Here's the drawing with two shaded views (mm, measured from the low corner). I have some questions. Give positions to 0.01 mm unless a question says otherwise; leave off trailing zeros. Write each loop counter-clockwise with the first axis right and the second up, starting at its lowest first coordinate (ties: lowest second). Pieces come first, ordered by that corner, then holes. Notation, with made-up numbers: M 18,24 L 49,24 A18 cw 49,43 Z; hole C -11.5,66.25 d1. An arc over 180 degrees is marked long. Answer as CSV lines item,"result". Start each with the question number.
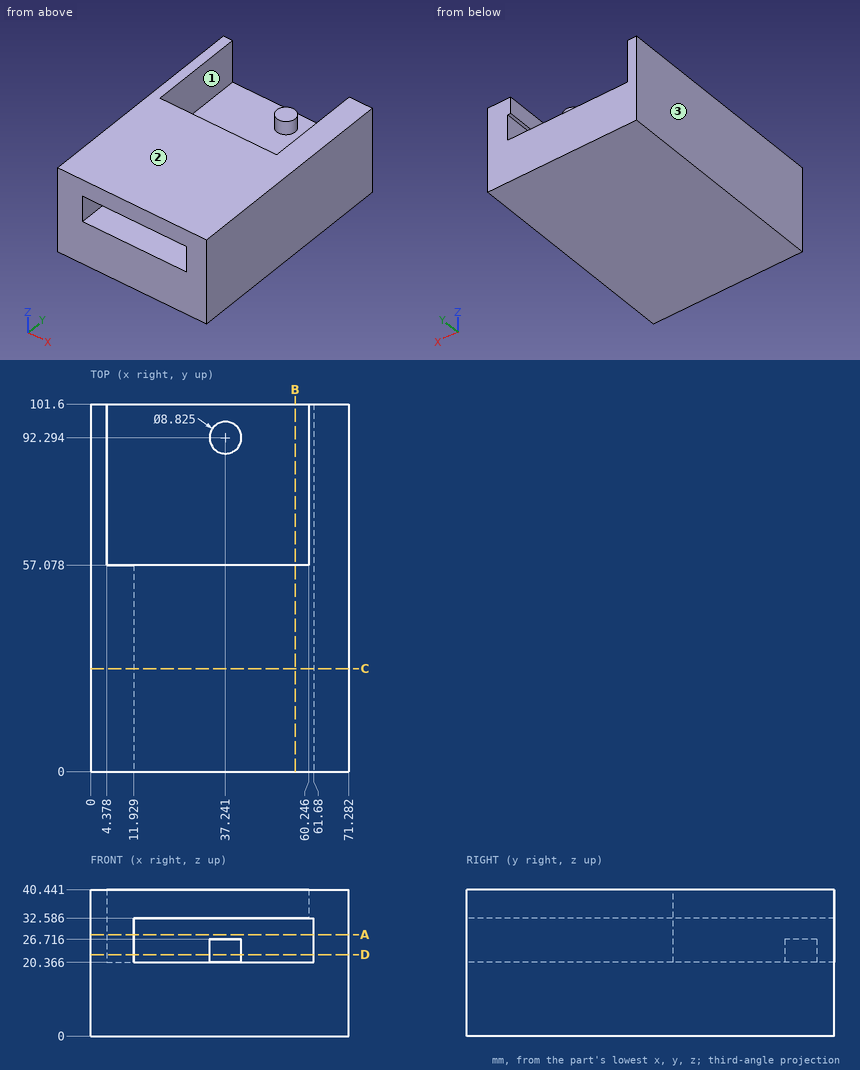
1. Imagine slicing it at C-C, the plane y = 28.5. Please give me the cut outline in (x, z).
2. Imagine slicing it at D-D, the plane z = 22.5. Please give me the cut outline in (x, y) (1 decimal).
3. Thinking about a two-plate mould opening in X: for the marked faces 1, 2 and 3, which applies, pulls with the +X half, pulls with the -X half, needs draft (parallel to the pull), parting line crosses it, or undercut?
4. Imagine slicing it at B-B, the plane x = 56.5. Please give me the cut outline in (y, z), plus the area to 3 significant figures.
5. Will this pin go through, and if not, where does the flat tip stop? P1, Ø4.5, axis at x = 38.5, y = 90.5, coming from the +Z side.
6. Imagine slicing it at A-A, the plane z = 28. Please give me the cut outline in (x, y).
7. Please list where these lines run through material, in increasing order: line 1 (Z direction, x = 42, y = 26); line 2 (X direction, y = 57, z = 29); line 3 (X direction, y = 70.5, z = 30).
Solutions:
1,outline,"M 0,0 L 71.28,0 L 71.28,40.44 L 0,40.44 Z; hole M 11.93,20.37 L 61.68,20.37 L 61.68,32.59 L 11.93,32.59 Z"
2,outline,"M 0,0 L 11.9,0 L 11.9,57.1 L 4.4,57.1 L 4.4,101.6 L 0,101.6 Z; C 37.2,92.3 d8.8; M 61.7,0 L 71.3,0 L 71.3,101.6 L 61.7,101.6 Z"
3,face 1,"undercut"
3,face 2,"needs draft"
3,face 3,"pulls with the -X half"
4,outline,"M 0,0 L 101.6,0 L 101.6,20.37 L 0,20.37 Z; M 0,32.59 L 57.08,32.59 L 57.08,40.44 L 0,40.44 Z"
4,area,"2,520 mm²"
5,P1,"z = 26.72"
6,outline,"M 0,0 L 11.93,0 L 11.93,57.08 L 4.38,57.08 L 4.38,101.6 L 0,101.6 Z; M 61.68,0 L 71.28,0 L 71.28,101.6 L 61.68,101.6 Z"
7,line 1,"0 to 20.37, 32.59 to 40.44"
7,line 2,"0 to 11.93, 61.68 to 71.28"
7,line 3,"0 to 4.38, 61.68 to 71.28"
